Read the model definition and answer for the solid it produces. Units are mm, in the model's axes. A direction names the side the tool comes from. Coordinates: 2 decimals unless noted, no trailing zeros. Loops run counter-clockwise (first coordinate to the right, second up) from the corner with the lowest first, then second, coordinate; pieces in that order, holes last. Notation, with made-up numbers: (46.5, 12) - (57.5, 12) arc R20 ccw to (57.5, 40) - close; hole circle Ø4 at (7, 61.25). An arc over 180 degrees is marked (long way). Use one line per item in the form item = value. Start each with the question number.
1) A cutting plane is placed at B-B (x = 0). Give the vertices of the cut face in (y, z).
2) A cutting plane is placed at D-D (y = -6). Give the vertices of the cut face in (x, z), and give its area (3 significant figures).
3) A cutting plane is placed at C-C (z = 9.5). Give the vertices of the cut face in (x, y), and give its area (3 significant figures).
4) Each of these flat-tipped pins is pushed along its axis until it touches: P1, Ø10, axis at y = 6.5, z = 16, coming from the -X side; P2, Ø4, axis at y = 25, z = 9.5, coming from the +X side; P3, Ø2, axis at y = 13.5, z = 17, coming from the -X side; P4, Ø1, axis at x = 11.5, y = 11, coming from the +Z side. Where does it stop, or does it pass through?
5) The mould has two halves that part along X. Classify faces 4 (the face through (13.91, -9.5, 12.68)), 5 (the face through (-16, -10, 12)), 6 (the face through (11.68, 16.69, 12.68)): released by +X, released by -X, zero draft, split by the parting line, or undercut.
6) Consider line 1 (X direction, y = 0, z = 14.5); line 2 (Y direction, x = 0.5, z = 17.25); line 3 (X direction, y = 27.5, z = 21.75). Determine where each line is inside the solid, lowest interval first.
7) A cutting plane is placed at A-A (y = 2). Give the vertices of the cut face in (x, z).
8) Which of the six approach directions +Z, -Z, +X, -X, +Y, -Y give full straight-line access (tool end or side, diameter ignored) to faces 1 (the face through (-13.896, -9.477, 12.675)), 2 (the face through (11.241, 25, 12)), 3 (the face through (-11.241, 25, 12))?
from build123d import *

# Parameters (mm, degrees)
F1_DEPTH = 25
F3_DEPTH = 25
F4_R     = 1
F5_R     = 5


with BuildPart() as f1:
    # F0 (on Top) → F1 (new body)
    with BuildSketch(Plane.XY):
        with BuildLine():
            ThreePointArc((-12.8720627718, -10), (0, 16.3), (12.8720627718, -10))
            Line((12.8720627718, -10), (17.089177862, -10))
            ThreePointArc((17.089177862, -10), (0, 19.8), (-17.089177862, -10))
            Line((-17.089177862, -10), (-12.8720627718, -10))
        make_face()
    extrude(amount=F1_DEPTH)

    # F2 (on face) → F3 (join, through all)
    with BuildSketch(Plane(origin=(0, 0, 0), x_dir=(1, 0, 0), z_dir=(0, 0, -1))):
        Polygon((11.2405515879, -16.3), (0, -16.3), (-11.2405515879, -16.3), (-11.2405515879, -36.3), (11.2405515879, -36.3), align=None)
    extrude(amount=-F3_DEPTH)

    # F4
    f4_edges = [f1.edges().sort_by_distance(p)[0] for p in [
        (-12.872063, -10, 12.5),
        (12.872063, -10, 12.5),
        (-17.089178, -10, 12.5),
        (17.089178, -10, 12.5),
    ]]
    fillet(f4_edges, radius=F4_R)

    # F5
    f5_edges = [f1.edges().sort_by_distance(p)[0] for p in [
        (-11.240552, 16.3, 12.5),
        (11.240552, 16.3, 12.5),
        (-11.240552, 36.3, 12.5),
        (11.240552, 36.3, 12.5),
    ]]
    fillet(f5_edges, radius=F5_R)


solid = f1.part
Found:
q1.outline = (16.3, 0) - (36.3, 0) - (36.3, 25) - (16.3, 25) - close
q2.outline = (-18.87, 0) - (-15.16, 0) - (-15.16, 25) - (-18.87, 25) - close; (15.16, 0) - (18.87, 0) - (18.87, 25) - (15.16, 25) - close
q2.area = 186 mm^2
q3.outline = (-17.38, -9.48) arc R1 ccw to (-16.51, -10) - (-14.77, -10) arc R1 ccw to (-13.92, -8.48) arc R16.3 cw (long way) to (13.92, -8.48) arc R1 ccw to (14.77, -10) - (16.51, -10) arc R1 ccw to (17.38, -9.48) arc R19.8 ccw to (12.97, 14.96) arc R5 cw to (11.24, 18.74) - (11.24, 31.3) arc R5 ccw to (6.24, 36.3) - (-6.24, 36.3) arc R5 ccw to (-11.24, 31.3) - (-11.24, 18.74) arc R5 cw to (-12.97, 14.96) arc R19.8 ccw to start
q3.area = 658 mm^2
q4.P1 = -19.74
q4.P2 = 11.24
q4.P3 = -15.36
q4.P4 = 25
q5.face_4 = undercut
q5.face_5 = zero draft
q5.face_6 = released by +X
q6.line_1 = -19.8 to -16.3, 16.3 to 19.8
q6.line_2 = 16.29 to 36.3
q6.line_3 = -11.24 to 11.24
q7.outline = (-19.7, 0) - (-16.18, 0) - (-16.18, 25) - (-19.7, 25) - close; (16.18, 0) - (19.7, 0) - (19.7, 25) - (16.18, 25) - close
q8.face_1 = +Z, -Z
q8.face_2 = +Z, -Z, +X, +Y
q8.face_3 = +Z, -Z, -X, +Y
